```python
from build123d import *

# Parameters (mm, degrees)
SKETCH2_R          = 1.75
CUT_EXTRUDE1_DEPTH = 0.1
SKETCH4_W          = 0.225
SKETCH4_H          = 2.5
FILLET1_R          = 0.2


with BuildPart() as part:
    # Sketch1 → Revolve1 (revolve)
    with BuildSketch(Plane.XY):
        with BuildLine():
            Line((2, 7), (0, 7))
            Line((0, 7), (0, 0))
            Line((0, 0), (1.970115999, 0))
            ThreePointArc((1.970115999, 0), (1.997744783, 0.172945308), (1.985594939, 0.347661679))
            ThreePointArc((1.985594939, 0.347661679), (1.963952003, 0.504056499), (1.956717438, 0.661775925))
            Line((1.956717438, 0.661775925), (1.956717438, 0.788075836))
            ThreePointArc((1.956717438, 0.788075836), (1.963946646, 0.983958609), (1.985594939, 1.178775635))
            ThreePointArc((1.985594939, 1.178775635), (1.99639383, 1.275956871), (2, 1.373669737))
            Line((2, 1.373669737), (2, 7))
        make_face()
    revolve(axis=Axis((0, 7, 0), (0, -1, 0)))

    # Sketch2 → Cut-Extrude1 (cut)
    with BuildSketch(Plane(origin=(0, 7, 0), x_dir=(-1, 0, 0), z_dir=(0, 1, 0))):
        with Locations(Location((0, 0, 0), (0, 0, 270))):
            Circle(SKETCH2_R)
    extrude(amount=-CUT_EXTRUDE1_DEPTH, mode=Mode.SUBTRACT)

    # Sketch4 → Revolve2 (revolve)
    with BuildSketch(Plane(origin=(0, 0, 0), x_dir=(-1, 0, 0), z_dir=(0, 0, -1)), mode=Mode.PRIVATE) as revolve2_sk:
        with Locations((-0.8625, -1.25)):
            Rectangle(SKETCH4_W, SKETCH4_H)
    revolve2 = revolve(revolve2_sk.sketch.rotate(Axis((0.75, -2.5, 0), (0, 1, 0)), 270), axis=Axis((0.75, -2.5, 0), (0, 1, 0)))

    # Fillet1
    fillet1_edges = [part.edges().sort_by_distance(p)[0] for p in [
        (-2, 7, 0),
        (-1.970115999, 0, 0),
    ]]
    fillet(fillet1_edges, radius=FILLET1_R)

    # Simetría3: Revolve2 across plane
    add(revolve2.mirror(Plane(origin=(0, 0, 0), x_dir=(0, 0, 1), z_dir=(1, 0, 0))))


solid = part.part
```
Read the model definition and answer for the solid it produces. Units are mm, in the model's axes. A direction names the side the tool comes from. Give positions to 0.01 mm unless a question says otherwise; leave off trailing zeros. Write each loop counter-clockwise with the first axis right and the second up, starting at its lowest first coordinate (ties: lowest second). Pieces come first, ordered by that corner, then holes. Notation, with made-up numbers: (2.25, 71.25) -> (40.25, 71.25) arc R15 cw to (40.25, 87.25) -> close; hole circle Ø8 at (64.25, 7.5). An arc over 180 degrees is marked (long way). Answer as a JSON object with one key per item and string values.
1) A tool of negligible diameter and unlimited length cuts with its end or side. For faces 1 (the cylindrical face through (0, 4, -2)), 2 (the flat face through (0, 6.9, 0)), from which of +Z, -Z, +X, -X, +Y, -Y can it reach the whole face along a straight path? Write none if from no direction.
Findings below:
{"face 1": "+Y, -Y", "face 2": "+Y"}
2) Section A-A on y = 3 is taken. Write down the section's boundary in (x, z), then the cut area to 3 significant figures.
Findings below:
{"outline": "circle Ø4 at (0, 0)", "area": "12.6 mm^2"}
3) Straight lines are drawn through the part: probe 1 along Y at (x, z) = (1.3, 1.1); probe 2 along X at (y, z) = (2, 0.1); probe 3 along Z at (x, y) = (0.25, 6.25). For each, find the intervals that lie inside material, in ascending order. Write a range as from..to.
Findings below:
{"probe 1": "y = 0..6.9", "probe 2": "x = -2..2", "probe 3": "z = -1.98..1.98"}
4) Flat-ended cylindrical pins translate along their axes: pin 1 Ø2 at (x, y) = (-1.5, 2.5) entering from -Z; pin 2 Ø1.5 at (x, z) = (0.5, -1.5) entering from -Y. Find the tip coordinate at first contact, or state that the pin passes through.
Findings below:
{"pin 1": "stops at z = -1.94", "pin 2": "stops at y = 0"}
